Input: dimensioned drawing with shaded views. Units: mm. Origin: part minimum x, y, z. A direction names the side the tool comes from. Coordinates: 2 decimals unless noted, no trailing zeros. Write each loop counter-clockwise with the first axis right and the second up, starting at its lowest first coordinate (ties: lowest second). Pieces come first, ordered by that corner, then holes. Notation, with made-up numbers: (7, -2.75) - (11, -2.75) arc R8 ccw to (11, 1.25) - close; hole circle Ø6 at (66.5, 13.5). An arc over 180 degrees is marked (long way). One line per question, with ' | ' between items.
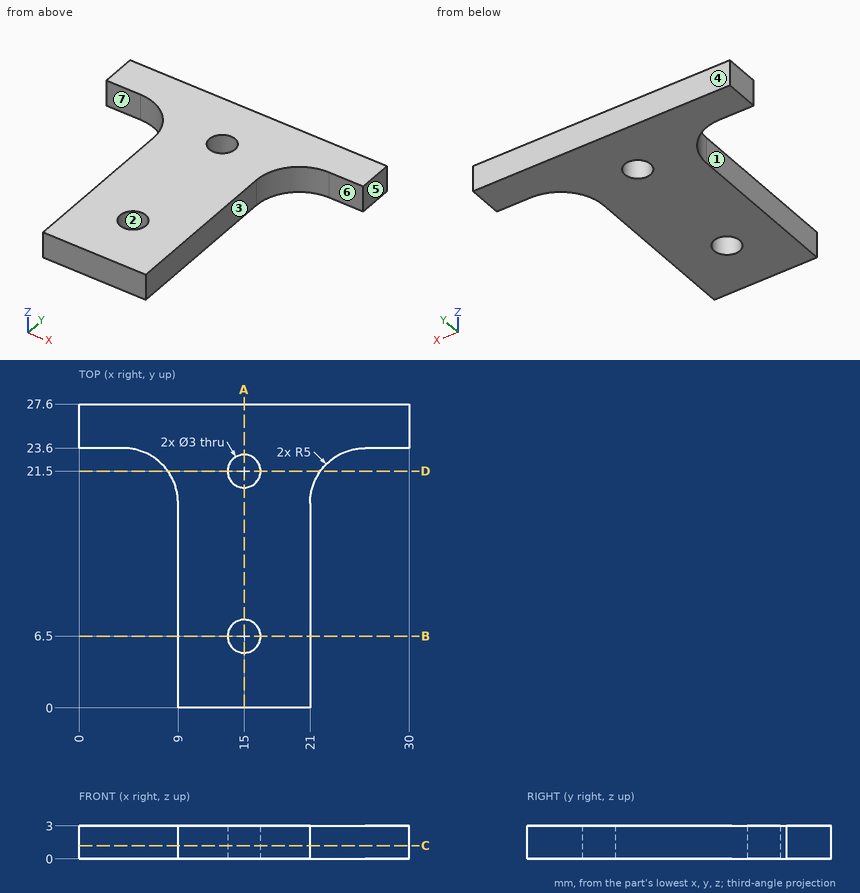
Item 1: Cut plane D-D on y = 21.5. Return loops of the section in (x, z), and give its area (3 significant figures).
Check sheet entries:
outline: (8.07, 0) - (13.5, 0) - (13.5, 3) - (8.07, 3) - close; (16.5, 0) - (21.93, 0) - (21.93, 3) - (16.5, 3) - close | area: 32.6 mm²
Item 2: Mould query, pull axis X, two halves, no side actions, for the marked faces 1, 2, 3 and 4. Classes: pulls with the +X half, pulls with the -X half, needs draft (parallel to the pull), parting line crosses it, or undercut.
Check sheet entries:
face 1: pulls with the -X half | face 2: undercut | face 3: pulls with the +X half | face 4: needs draft
Item 3: Pin query (flat end, axial travel): pin 1 Ø1.5 at (x, z) = (2, 2) entering from -Y. Return the tip coordinate at first contact, or that it passes through.
Check sheet entries:
pin 1: y = 23.6
Item 4: Ray query, line 1 along Y through (x, z) = (15, 1.5); line 2 along Y through (x, z) = (26, 2.4); line 3 along X through (y, z) = (3.25, 0.9). Return the intervals inside material, ascending. Write a range as [from, to].
Check sheet entries:
line 1: [0, 5], [8, 20], [23, 27.6] | line 2: [23.6, 27.6] | line 3: [9, 21]
Item 5: Cut plane B-B on y = 6.5. Return loops of the section in (x, z), and give its area (3 significant figures).
Check sheet entries:
outline: (9, 0) - (13.5, 0) - (13.5, 3) - (9, 3) - close; (16.5, 0) - (21, 0) - (21, 3) - (16.5, 3) - close | area: 27.0 mm²
Item 6: Cut plane A-A on x = 15. Return loops of the section in (y, z), and give its area (3 significant figures).
Check sheet entries:
outline: (0, 0) - (5, 0) - (5, 3) - (0, 3) - close; (8, 0) - (20, 0) - (20, 3) - (8, 3) - close; (23, 0) - (27.6, 0) - (27.6, 3) - (23, 3) - close | area: 64.8 mm²
Item 7: Cut plane C-C on z = 1.2. Return loops of the section in (x, y).
Check sheet entries:
outline: (0, 23.6) - (4, 23.6) arc R5 cw to (9, 18.6) - (9, 0) - (21, 0) - (21, 18.6) arc R5 cw to (26, 23.6) - (30, 23.6) - (30, 27.6) - (0, 27.6) - close; hole circle Ø3 at (15, 6.5); hole circle Ø3 at (15, 21.5)
Item 8: Access query for the marked faces 5, 6 and 7. Directions: +Z, -Z, +X, -X, +Y, -Y. A direction counts if a zero-diameter tool reaches every point of the face in a straight line with its end or side. Return the directions, or none.
Check sheet entries:
face 5: +Z, -Z, +X, +Y, -Y | face 6: +Z, -Z, +X, -Y | face 7: +Z, -Z, -X, -Y
